Autodesk Inventor part; units mm, degrees
ref_plane "YZ Plane" through (0, 0, 0) normal (1, 0, 0) x (0, 1, 0)
ref_plane "XZ Plane" through (0, 0, 0) normal (0, 1, 0) x (-1, 0, 0)
ref_plane "XY Plane" through (0, 0, 0) normal (0, 0, 1) x (1, 0, 0)
sketch "Skizze1" plane through (0, 0, 0) normal (0, 0, 1) x (1, 0, 0)
  line L0 (-19, -11) -> (-19, -7)
  line L1 (-19, -7) -> (-15.8989, -7)
  line L2 (-15.8989, -7) -> (-14.5, -4)
  line L3 (-14.5, -4) -> (-14.5, 0)
  line L4 (-14.5, 0) -> (14.5, 0)
  line L5 (14.5, 0) -> (14.5, -4)
  line L6 (14.5, -4) -> (15.8989, -7)
  line L7 (15.8989, -7) -> (19, -7)
  line L8 (19, -7) -> (19, -11)
  line L9 (19, -11) -> (25, -17)
  line L10 (25, -17) -> (29, -17)
  line L11 (29, -17) -> (29, 20)
  line L12 (29, 20) -> (-29, 20)
  line L13 (-29, 20) -> (-29, -17)
  line L14 (-29, -17) -> (-25, -17)
  line L15 (-25, -17) -> (-19, -11)
  line L16 (0, 0) -> (0, -29.3821)
  dimension "d5" = 29
  dimension "d6" = 20
  dimension "d7" = 4
  dimension "d8" = 4.5
  dimension "d10" = 38
  dimension "d12" = 25
  dimension "d13" = 10
  dimension "d14" = 10
  dimension "d15" = 7
  dimension "d16" = 45
  dimension "d17" = 10
  dimension "d18" = 4
extrude "Extrusion1" add sketch "Skizze1" along normal mid plane 10
sketch "Skizze2" plane through (25, -17, 5) normal (0, -1, 0) x (1, 0, 0)
  line L0 (4, -10) -> (4, 0)
  line L1 (-54, -10) -> (4, -10)
  line L2 (4, 0) -> (-6, 0)
  line L3 (-6, 0) -> (-6, -10)
  line L4 (-6, -10) -> (4, -10)
  line L5 (4, -10) -> (4, 0)
  point P0 (-25, -5)
  dimension "d21" = 10
extrude "Extrusion2" cut sketch "Skizze2" against normal blind 10
properties part number "_WT_Aufnahme_Antriebseinheit3"
The listing builds one solid part. Answer for the finished solid, in the listing's coordinates (mm). A direction names the side the tool comes from. Give positions to 0.01 mm unless a question says otherwise; leave off trailing zeros. Order: outer loops, then holes, each group sorted by start corner. A loop starts at its lowest first (then second) coordinate and runs counter-clockwise, first axis right, second up. Notation, with made-up numbers: (42.5, -11) - (99.5, -11) arc R12 cw to (99.5, 9) - close; hole circle Ø2 at (34, -37.5). An arc over 180 degrees is marked (long way). Answer in a Markdown table with one row per item. Add a question column.
Q1. For a pull along X with two mould halves and no side action, classify faces 4 (the flat face through (14.5, -2, 0)), 5 (the flat face through (-29, 2, 0)), 6 (the flat face through (-22, -14, 0)), 7 (the flat face through (0, 6, -5)) as released by +X, released by -X, zero draft, split by the parting line, or undercut.
Q2. Which of the six approach directions +Z, -Z, +X, -X, +Y, -Y give full straight-line access (tool end or side, diameter ignored) to faces 1 (the flat face through (-19, -9, 0)), 2 (the flat face through (29, 6, 0)), 3 (the flat face through (-15.2, -5.5, -0.1))?
Q3. The part is cut by section D-D (x = 23). Determine the outline of the cut face in (y, z).
Q4. The part is cut by section A-A (y = -2.5). Determine the outline of the cut face in (x, z), then the cut area to 3 significant figures.
Q5. Given P1, Ø1.2, axis at y = -8.5, z = 1.5, coming from the +X side; P2, Ø0.9, axis at x = -17, z = 2, coming from the -Y side, each flat-ended and moving along its own axis, determine where each tip first touches the part or whether it passes through.
Q6. Find the intervals of material crossed by line 1 along X through (y, z) = (-3.5, 1); line 2 along Y through (x, z) = (-18.5, 2.75); line 3 along Y through (x, z) = (-1, 0.75), in increasing order. Write a range as [from, to].
Q7. The part is cut by section C-C (x = -7). Determine the outline of the cut face in (y, z).
Q8. The part is cut by section B-B (z = -0.25). Determine the outline of the cut face in (x, y).
Determined:
| question | item | result |
|---|---|---|
| 1 | face 4 | undercut |
| 1 | face 5 | released by -X |
| 1 | face 6 | released by +X |
| 1 | face 7 | zero draft |
| 2 | face 1 | +Z, -Z, +X, -Y |
| 2 | face 2 | +Z, -Z, +X, +Y, -Y |
| 2 | face 3 | +Z, -Z, -Y |
| 3 | outline | (-7, -5) - (20, -5) - (20, 5) - (-7, 5) - close |
| 4 | outline | (-29, -5) - (-14.5, -5) - (-14.5, 5) - (-29, 5) - close; (14.5, -5) - (29, -5) - (29, 5) - (14.5, 5) - close |
| 4 | area | 290 mm² |
| 5 | P1 | stops at x = -19 |
| 5 | P2 | stops at y = -7 |
| 6 | line 1 | x = [-29, -14.5], [14.5, 29] |
| 6 | line 2 | y = [-7, 20] |
| 6 | line 3 | y = [0, 20] |
| 7 | outline | (0, -5) - (20, -5) - (20, 5) - (0, 5) - close |
| 8 | outline | (-29, -17) - (-25, -17) - (-19, -11) - (-19, -7) - (-15.9, -7) - (-14.5, -4) - (-14.5, 0) - (14.5, 0) - (14.5, -4) - (15.9, -7) - (29, -7) - (29, 20) - (-29, 20) - close |
